Check sheet for the drawn part. Datum: minimum x, y, z corner. Units: mm. Give positions to 0.01 mm unless a question says otherwise; leave off trailing zeros. Loops run counter-clockwise (first coordinate to the right, second up) from the corner with the lowest first, then second, coordinate; pieces in that order, holes last.
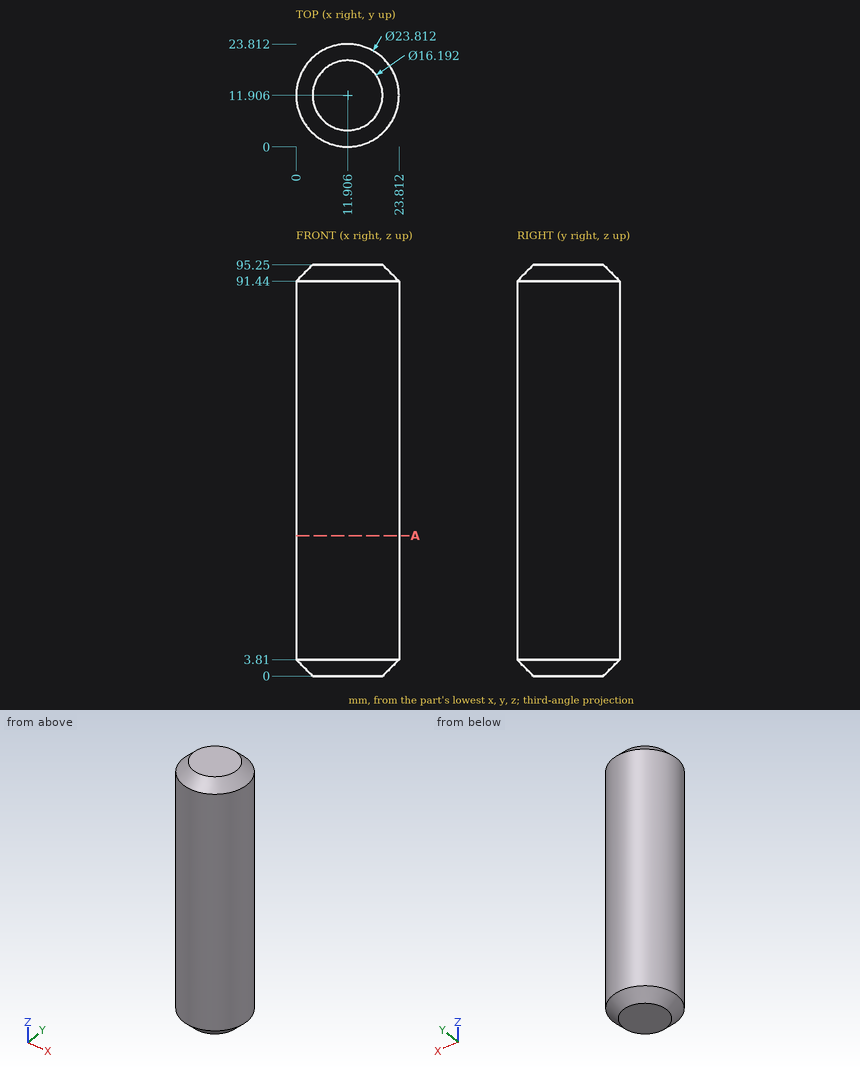
(1) Section check A-A on z = 32.5. Record the boundary of the cut face in (x, y), plus the area to 3 significant figures.
(2) Gauge pin test, flat ends, axial feed: pin 1 Ø2 at (x, z) = (10, 58) entering from -Y; pin 2 Ø3 at (x, z) = (15.5, 54.5) entering from +Y; pin 3 Ø6 at (x, z) = (20, 79.5) entering from -Y; pin 4 Ø5 at (y, z) = (13, 55.5) entering from +X. Record the tip position at first contact, or that the pin passes through.
(3) Material ranges on line 1 (X direction, y = 12.5, z = 30); line 2 (Z direction, x = 14.5, y = 20); line 3 (Z direction, x = 15.5, y = 1.75), recorded low to high.
Computed values:
1. outline: circle Ø23.81 at (11.91, 11.91)
1. area: 445 mm2
2. pin 1: stops at y = 0.03
2. pin 2: stops at y = 23.63
2. pin 3: stops at y = 1.14
2. pin 4: stops at x = 23.81
3. line 1: x = 0.01 to 23.8
3. line 2: z = 0.4 to 94.85
3. line 3: z = 2.68 to 92.57
